from build123d import *

# Parameters (mm, degrees)
SKETCH1_W           = 152.4
SKETCH1_H           = 114.3
SKETCH1_R           = 10.287
BOSS_EXTRUDE1_DEPTH = 12.7
EXTRUDE_THIN1_DEPTH = 63.5
SKETCH1_4_R         = 10.287
SKETCH1_4_R_2       = 5.08
BOSS_EXTRUDE2_DEPTH = 12.7
SKETCH1_5_R         = 10.287
SKETCH1_5_R_2       = 5.08
CUT_EXTRUDE1_DEPTH  = 6.35


with BuildPart() as part:
    # Sketch1 → Boss-Extrude1 (new body)
    with BuildSketch(Plane(origin=(0, 0, 0), x_dir=(1, 0, 0), z_dir=(0, 1, 0))):
        Rectangle(SKETCH1_W, SKETCH1_H)
        with Locations((-50.8, 31.75)):
            Circle(SKETCH1_R, mode=Mode.SUBTRACT)
        with Locations((50.8, 31.75)):
            Circle(SKETCH1_R, mode=Mode.SUBTRACT)
        with Locations((50.8, -31.75)):
            Circle(SKETCH1_R, mode=Mode.SUBTRACT)
        with Locations((-50.8, -31.75)):
            Circle(SKETCH1_R, mode=Mode.SUBTRACT)
        with BuildLine():
            ThreePointArc((25.4, -12.7), (38.1, 0), (25.4, 12.7))
            Line((25.4, 12.7), (-25.4, 12.7))
            ThreePointArc((-25.4, 12.7), (-38.1, 0), (-25.4, -12.7))
            Line((-25.4, -12.7), (25.4, -12.7))
        make_face(mode=Mode.SUBTRACT)
    extrude(amount=-BOSS_EXTRUDE1_DEPTH)

    # Sketch1<3> → Extrude-Thin1 (add)
    with BuildSketch(Plane(origin=(0, 0, 0), x_dir=(1, 0, 0), z_dir=(0, 1, 0))):
        with BuildLine():
            Line((25.4, -17.78), (-25.4, -17.78))
            ThreePointArc((-25.4, -17.78), (-43.18, 0), (-25.4, 17.78))
            Line((-25.4, 17.78), (25.4, 17.78))
            ThreePointArc((25.4, 17.78), (43.18, 0), (25.4, -17.78))
        make_face()
        with BuildLine():
            Line((25.4, -12.7), (-25.4, -12.7))
            ThreePointArc((-25.4, -12.7), (-38.1, 0), (-25.4, 12.7))
            Line((-25.4, 12.7), (25.4, 12.7))
            ThreePointArc((25.4, 12.7), (38.1, 0), (25.4, -12.7))
        make_face(mode=Mode.SUBTRACT)
    extrude(amount=EXTRUDE_THIN1_DEPTH)

    # Sketch1<4> → Boss-Extrude2 (add)
    with BuildSketch(Plane(origin=(0, 0, 0), x_dir=(1, 0, 0), z_dir=(0, 1, 0))):
        with Locations((-50.8, 31.75)):
            Circle(SKETCH1_4_R)
        with Locations((-50.8, 31.75)):
            Circle(SKETCH1_4_R_2, mode=Mode.SUBTRACT)
        with Locations((-50.8, -31.75)):
            Circle(SKETCH1_4_R)
        with Locations((-50.8, -31.75)):
            Circle(SKETCH1_4_R_2, mode=Mode.SUBTRACT)
        with Locations((50.8, -31.75)):
            Circle(SKETCH1_4_R)
        with Locations((50.8, -31.75)):
            Circle(SKETCH1_4_R_2, mode=Mode.SUBTRACT)
        with Locations((50.8, 31.75)):
            Circle(SKETCH1_4_R)
        with Locations((50.8, 31.75)):
            Circle(SKETCH1_4_R_2, mode=Mode.SUBTRACT)
    extrude(amount=-BOSS_EXTRUDE2_DEPTH)

    # Sketch1<5> → Cut-Extrude1 (cut)
    with BuildSketch(Plane(origin=(0, 0, 0), x_dir=(1, 0, 0), z_dir=(0, 1, 0))):
        with Locations((-50.8, -31.75)):
            Circle(SKETCH1_5_R)
        with Locations((-50.8, -31.75)):
            Circle(SKETCH1_5_R_2, mode=Mode.SUBTRACT)
        with Locations((-50.8, 31.75)):
            Circle(SKETCH1_5_R)
        with Locations((-50.8, 31.75)):
            Circle(SKETCH1_5_R_2, mode=Mode.SUBTRACT)
        with Locations((50.8, 31.75)):
            Circle(SKETCH1_5_R)
        with Locations((50.8, 31.75)):
            Circle(SKETCH1_5_R_2, mode=Mode.SUBTRACT)
        with Locations((50.8, -31.75)):
            Circle(SKETCH1_5_R)
        with Locations((50.8, -31.75)):
            Circle(SKETCH1_5_R_2, mode=Mode.SUBTRACT)
    extrude(amount=-CUT_EXTRUDE1_DEPTH, mode=Mode.SUBTRACT)


solid = part.part
Here's how the part is built. I have some questions about the finished solid (model axes, mm). A direction names the side the tool comes from. Give positions to 0.01 mm unless a question says otherwise; leave off trailing zeros. Loops run counter-clockwise (first coordinate to the right, second up) from the corner with the lowest first, then second, coordinate; pieces in that order, holes last. Notation, with made-up numbers: (62.5, -15) -> (82.5, -15) arc R23 ccw to (82.5, 23) -> close; hole circle Ø2 at (-18.5, -16). An arc over 180 degrees is marked (long way). Answer as a JSON object with one key per item and string values. Group by question number.
Item 1: Imagine slicing it at D-D on x = -50.8. Write out the boundary of the cut face in (y, z).
Item 2: Will these pins go through, and if not, where does the flat tip stop? pin 1 (16.5 mm diameter, centred on x = 55.5, z = -35, fed in from +Y); pin 2 (10.5 mm diameter, centred on x = -50, z = -30.5, fed in from +Y); pin 3 (5 mm diameter, centred on x = 3, y = 37.5, fed in from -Z).
Item 3: Imagine slicing it at B-B on z = 0. Write out the boundary of the cut face in (x, y), then the cut area to 3 significant figures.
Item 4: Imagine slicing it at A-A on x = 15. Write out the boundary of the cut face in (y, z), then the cut area to 3 significant figures.
Item 5: On a 3-axis mill with a long thin cutter (end or side, diameter ignored), from which of +Z, -Z, +X, -X, +Y, -Y can I reach the whole of each face in a straight line? I mean faces 4 (the flat face through (0, 25, 12.7)), 5 (the cylindrical face through (43.176, 31.306, -0.391)), 6 (the flat face through (-56, -6.35, 34)). Say none if no direction works.
Item 6: Imagine slicing it at C-C on y = 39.5. Write out the boundary of the cut face in (x, z), then the cut area to 3 significant figures.
Item 7: Thinking about a two-plate mould opening in Z: for faces 1 (the cylindrical face through (-43.176, 31.306, 0.391)), 2 (the cylindrical face through (-61.077, -3.131, -32.202)), 3 (the flat face through (0, 31, 17.78)), which applies, pulls with the +Z half, pulls with the -Z half, needs draft (parallel to the pull), parting line crosses it, or undercut?
Item 8: I need wall thicknesses on L1, parallel to Z at x = 50.8, y = -4; L2, parallel to Z at x = 50.8, y = -8.75; L3, parallel to X at y = -9.25, z = -31.75. Which ranges of each line are inside material? Lowest first, please.
Answer list:
{
 "1": {"outline": "(-12.7, -57.15) -> (0, -57.15) -> (0, -42.04) -> (-6.35, -42.04) -> (-6.35, -36.83) -> (-12.7, -36.83) -> close; (-12.7, -26.67) -> (-6.35, -26.67) -> (-6.35, -21.46) -> (0, -21.46) -> (0, 21.46) -> (-6.35, 21.46) -> (-6.35, 26.67) -> (-12.7, 26.67) -> close; (-12.7, 36.83) -> (-6.35, 36.83) -> (-6.35, 42.04) -> (0, 42.04) -> (0, 57.15) -> (-12.7, 57.15) -> close"},
 "2": {"pin 1": "stops at y = 0", "pin 2": "stops at y = -6.35", "pin 3": "stops at z = -17.78"},
 "3": {"outline": "(-76.2, -12.7) -> (-38.1, -12.7) -> (-38.1, 63.5) -> (-43.18, 63.5) -> (-43.18, 0) -> (-76.2, 0) -> close; (38.1, -12.7) -> (76.2, -12.7) -> (76.2, 0) -> (43.18, 0) -> (43.18, 63.5) -> (38.1, 63.5) -> close", "area": "1,610 mm2"},
 "4": {"outline": "(-12.7, -57.15) -> (0, -57.15) -> (0, -17.78) -> (63.5, -17.78) -> (63.5, -12.7) -> (-12.7, -12.7) -> close; (-12.7, 12.7) -> (63.5, 12.7) -> (63.5, 17.78) -> (0, 17.78) -> (0, 57.15) -> (-12.7, 57.15) -> close", "area": "1,770 mm2"},
 "5": {"face 4": "+Y, -Y", "face 5": "+X, +Y", "face 6": "+Y"},
 "6": {"outline": "(-25.4, -17.78) -> (25.4, -17.78) arc R17.78 ccw to (25.4, 17.78) -> (-25.4, 17.78) arc R17.78 ccw to start; hole (-25.4, -12.7) -> (25.4, -12.7) arc R12.7 ccw to (25.4, 12.7) -> (-25.4, 12.7) arc R12.7 ccw to start", "area": "1,000 mm2"},
 "7": {"face 1": "parting line crosses it", "face 2": "undercut", "face 3": "pulls with the +Z half"},
 "8": {"L1": "z = -57.15 to -42.04, -21.46 to 21.46, 42.04 to 57.15", "L2": "z = -57.15 to -36.83, -26.67 to 26.67, 36.83 to 57.15", "L3": "x = -76.2 to -55.88, -45.72 to 45.72, 55.88 to 76.2"}
}
